Part print with two shaded views. Sizes in mm from the minimum x, y, z corner. A direction names the side the tool comes from. Round coordinates to 2 decimals unless told otherwise and drop trailing zeros. Write each loop counter-clockwise with the first axis right and the second up, starting at its lowest first coordinate (ties: lowest second). Pieces come first, ordered by that corner, then holes.
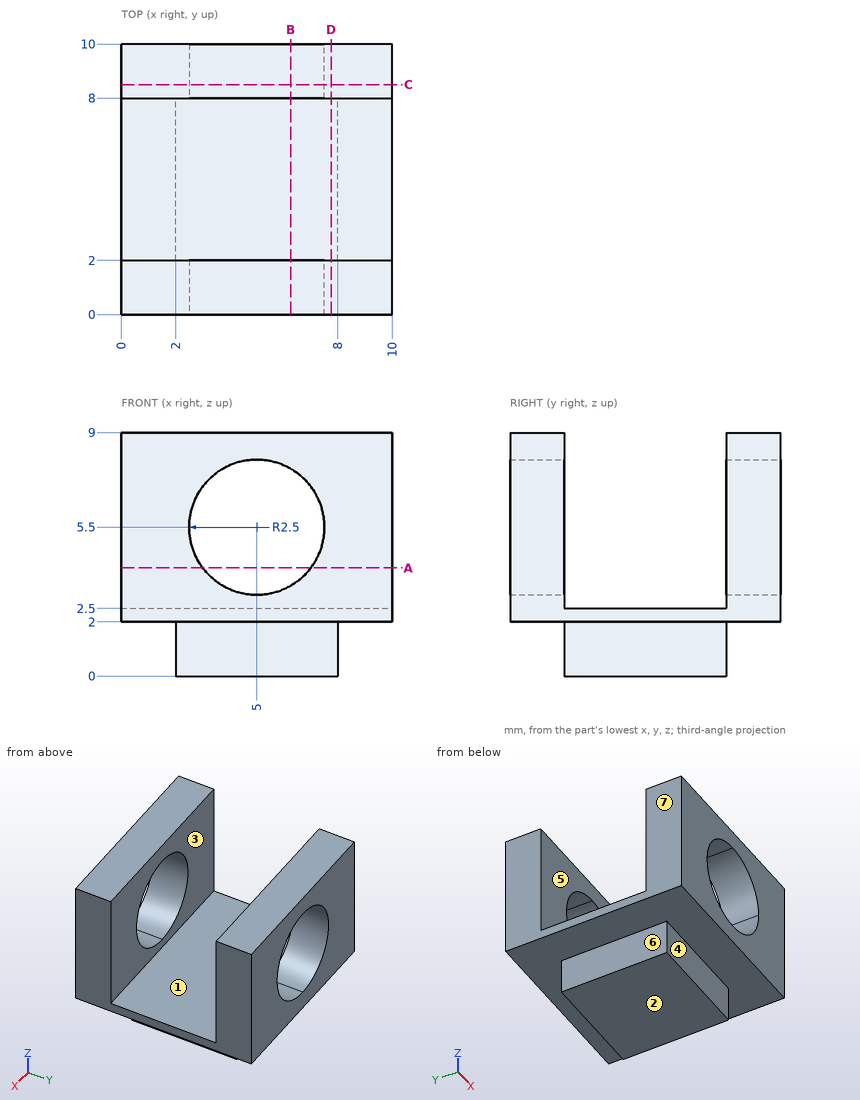
Q1. Cut at A-A on z = 4. Write the cut outline in (x, y), plus the area to 3 significant figures.
Values follow:
outline: (0, 0) - (3, 0) - (3, 2) - (0, 2) - close; (0, 8) - (3, 8) - (3, 10) - (0, 10) - close; (7, 0) - (10, 0) - (10, 2) - (7, 2) - close; (7, 8) - (10, 8) - (10, 10) - (7, 10) - close
area: 24.0 mm2
Q2. Mould opens along Y. For the marked faces 1, 2, 3 and 4 say: +Y half, -Y half, draft (parallel to the pull), parting line (faces both ways), or undercut.
Values follow:
face 1: undercut
face 2: draft
face 3: undercut
face 4: -Y half
Q3. Drop flat-ended pins along their axis: pin 1 (1.8 mm diameter, centred on x = 3, y = 5, fed in from +Z); pin 2 (4 mm diameter, centred on x = 3.5, y = 3.5, fed in from +Z); pin 3 (2 mm diameter, centred on y = 5.5, z = 0.5, fed in from -X); pin 4 (1 mm diameter, centred on x = 4.5, z = 1, fed in from -Y). Give the stop position or say it passes through.
Values follow:
pin 1: stops at z = 2.5
pin 2: stops at z = 9
pin 3: stops at x = 2
pin 4: stops at y = 2
Q4. Cut at D-D on x = 7.75. Write the cut outline in (y, z).
Values follow:
outline: (0, 2) - (2, 2) - (2, 0) - (8, 0) - (8, 2) - (10, 2) - (10, 9) - (8, 9) - (8, 2.5) - (2, 2.5) - (2, 9) - (0, 9) - close
Q5. Which spindle directions (+Z, -Z, +X, -X, +Y, -Y) get a long thin tool onto all of the face, cutting with end or side? Do the marked faces 5, 6 and 7. Say none if no direction does.
Values follow:
face 5: +Z, +X, -X
face 6: -Z, -X, +Y, -Y
face 7: +Z, -Z, -X, +Y, -Y
Q6. Cut at C-C on y = 8.5. Write the cut outline in (x, z).
Values follow:
outline: (0, 2) - (10, 2) - (10, 9) - (0, 9) - close; hole circle Ø5 at (5, 5.5)
Q7. Wall check: L1, parallel to Y at x = 3, z = 3.5; L2, parallel to Z at x = 0.75, y = 6.75; L3, parallel to X at y = 5.5, z = 0.5. Give the ranges that are in metal, low to high.
Values follow:
L1: y = 0 to 2, 8 to 10
L2: z = 2 to 2.5
L3: x = 2 to 8
Q8. Cut at B-B on x = 6.25. Write the cut outline in (y, z), plus the area to 3 significant figures.
Values follow:
outline: (0, 2) - (2, 2) - (2, 0) - (8, 0) - (8, 2) - (10, 2) - (10, 3.33) - (8, 3.33) - (8, 2.5) - (2, 2.5) - (2, 3.33) - (0, 3.33) - close; (0, 7.67) - (2, 7.67) - (2, 9) - (0, 9) - close; (8, 7.67) - (10, 7.67) - (10, 9) - (8, 9) - close
area: 25.7 mm2
